Build history of the part. All positions in model axes, mm. A direction names the side the tool comes from. Give positions to 0.01 mm unless a question says otherwise; leave off trailing zeros. Order: outer loops, then holes, each group sorted by start corner. A loop starts at its lowest first (then second) coordinate and runs counter-clockwise, first axis right, second up. Notation, with made-up numbers: M 84,30.25 L 133,30.25 A23 ccw 133,58.25 Z; hole C -16,40 d10. An arc over 180 degrees is marked long. Answer as CSV lines item,"result".
from build123d import *

# Parameters (mm, degrees)
SKETCH_1_W          = 40
SKETCH_1_H          = 20
EXTRUDE_1_DEPTH     = 37
SKETCH_2_W          = 54
SKETCH_2_H          = 20
EXTRUDE_2_DEPTH     = 2.5
SKETCH_3_R          = 2.2
CUT_EXTRUDE_1_DEPTH = 2.5
SKETCH_5_W          = 1.5
SKETCH_5_H          = 2.2
CUT_EXTRUDE_2_DEPTH = 2.5
FILLET_1_R          = 2
EXTRUDE_3_DEPTH     = 2
SKETCH_7_R          = 7.5
EXTRUDE_4_DEPTH     = 1.5
SKETCH_8_R          = 5.5
EXTRUDE_5_DEPTH     = 0.5
SKETCH_9_R          = 3
EXTRUDE_6_DEPTH     = 4
SKETCH_10_R         = 1.5
CUT_EXTRUDE_3_DEPTH = 5


with BuildPart() as part:
    # 草图1 → 凸台-拉伸1 (new body)
    with BuildSketch(Plane(origin=(0, 0, 0), x_dir=(1, 0, 0), z_dir=(0, 1, 0))):
        Rectangle(SKETCH_1_W, SKETCH_1_H)
    extrude(amount=EXTRUDE_1_DEPTH)

    # 草图2 → 凸台-拉伸2 (add)
    with BuildSketch(Plane(origin=(0, 29, 0), x_dir=(-1, 0, 0), z_dir=(0, -1, 0))):
        Rectangle(SKETCH_2_W, SKETCH_2_H)
    extrude(amount=-EXTRUDE_2_DEPTH)

    # 草图3 → 切除-拉伸1 (cut)
    with BuildSketch(Plane(origin=(0, 29, 0), x_dir=(-1, 0, 0), z_dir=(0, -1, 0))):
        with Locations(Location((24.2, 5, 0), (0, 0, 90))):
            Circle(SKETCH_3_R)
        with Locations(Location((-24.2, 5, 0), (0, 0, 90))):
            Circle(SKETCH_3_R)
        with Locations(Location((24.2, -5, 0), (0, 0, 90))):
            Circle(SKETCH_3_R)
        with Locations(Location((-24.2, -5, 0), (0, 0, 90))):
            Circle(SKETCH_3_R)
    extrude(amount=-CUT_EXTRUDE_1_DEPTH, mode=Mode.SUBTRACT)

    # 草图5 → 切除-拉伸2 (cut)
    with BuildSketch(Plane(origin=(0, 29, 0), x_dir=(-1, 0, 0), z_dir=(0, -1, 0))):
        with Locations((-26.25, 5)):
            Rectangle(SKETCH_5_W, SKETCH_5_H)
        with Locations((26.25, 5)):
            Rectangle(SKETCH_5_W, SKETCH_5_H)
        with Locations((26.25, -5)):
            Rectangle(SKETCH_5_W, SKETCH_5_H)
        with Locations((-26.25, -5)):
            Rectangle(SKETCH_5_W, SKETCH_5_H)
    extrude(amount=-CUT_EXTRUDE_2_DEPTH, mode=Mode.SUBTRACT)

    # 圆角1
    fillet_1_edges = [part.edges().sort_by_distance(p)[0] for p in [
        (27, 30.25, -10),
        (-27, 30.25, 10),
        (27, 30.25, 10),
        (-27, 30.25, -10),
    ]]
    fillet(fillet_1_edges, radius=FILLET_1_R)

    # 草图6 → 凸台-拉伸3 (add)
    with BuildSketch(Plane(origin=(0, 37, 0), x_dir=(1, 0, 0), z_dir=(0, 1, 0))):
        with BuildLine():
            Line((-10, 9), (15, 9))
            Line((15, 9), (15, -9))
            Line((15, -9), (-10, -9))
            ThreePointArc((-10, -9), (-19, 0), (-10, 9))
        make_face()
    extrude(amount=EXTRUDE_3_DEPTH)

    # 草图7 → 凸台-拉伸4 (add)
    with BuildSketch(Plane(origin=(0, 39, 0), x_dir=(1, 0, 0), z_dir=(0, 1, 0))):
        with Locations(Location((-10, 0, 0), (0, 0, 270))):
            Circle(SKETCH_7_R)
    extrude(amount=EXTRUDE_4_DEPTH)

    # 草图8 → 凸台-拉伸5 (add)
    with BuildSketch(Plane(origin=(0, 40.5, 0), x_dir=(1, 0, 0), z_dir=(0, 1, 0))):
        with Locations(Location((-10, 0, 0), (0, 0, 270))):
            Circle(SKETCH_8_R)
    extrude(amount=EXTRUDE_5_DEPTH)

    # 草图9 → 凸台-拉伸6 (add)
    with BuildSketch(Plane(origin=(0, 41, 0), x_dir=(1, 0, 0), z_dir=(0, 1, 0))):
        with Locations(Location((-10, 0, 0), (0, 0, 270))):
            Circle(SKETCH_9_R)
    extrude(amount=EXTRUDE_6_DEPTH)

    # 草图10 → 切除-拉伸3 (cut)
    with BuildSketch(Plane(origin=(0, 45, 0), x_dir=(1, 0, 0), z_dir=(0, 1, 0))):
        with Locations(Location((-10, 0, 0), (0, 0, 270))):
            Circle(SKETCH_10_R)
    extrude(amount=-CUT_EXTRUDE_3_DEPTH, mode=Mode.SUBTRACT)


solid = part.part
Item 1: 3-axis set-ups, long thin cutter, end or side, ignore diameter. For faces 1 (the cylindrical face through (-17.32, 39.74, -1.63)), 2 (the flat face through (15, 38, 0)), 3 (the cylindrical face through (-22, 30, -5)): which of +Z, -Z, +X, -X, +Y, -Y reach the whole face in a straight line?
Geometry says:
face 1,"+Y"
face 2,"+Z, -Z, +X, +Y"
face 3,"+Y, -Y"
Item 2: Pull direction Z, two halves, no side cores. Call faces 4 (the cylindrical face through (26.43, 30.27, 9.4)), 5 (the cylindrical face through (22, 30, -5)), 6 (the flat face through (-27, 30, 0)): released by +Z, released by -Z, zero draft, split by the parting line, or undercut.
Geometry says:
face 4,"released by +Z"
face 5,"undercut"
face 6,"zero draft"
Item 3: Band-saw the part on B-B (x = 0). Give the cut face in (y, z), and give its area (3 significant figures).
Geometry says:
outline,"M 0,-10 L 37,-10 L 37,-9 L 39,-9 L 39,9 L 37,9 L 37,10 L 0,10 Z"
area,"776 mm2"
Item 4: Band-saw the part on A-A (x = -24.2). Give the cut face in (y, z), and give its area (3 significant figures).
Geometry says:
outline,"M 29,-10 L 31.5,-10 L 31.5,-7.2 L 29,-7.2 Z; M 29,-2.8 L 31.5,-2.8 L 31.5,2.8 L 29,2.8 Z; M 29,7.2 L 31.5,7.2 L 31.5,10 L 29,10 Z"
area,"28.0 mm2"
Item 5: Probe line 1 along Z through (x, y) = (24, 30); line 2 along X through (y, z) = (43.3, 0); line 3 along X through (y, z) = (29.9, -5). List the from-to ranges inside material, lowest first. Write a range as from..to.
Geometry says:
line 1,"z = -10..-7.19, -2.81..2.81, 7.19..10"
line 2,"x = -13..-11.5, -8.5..-7"
line 3,"x = -22..22"
Item 6: Drop flat-ended pins along their axis: pin 1 (6 mm diameter, centred on y = 14.5, z = 6.5, fed in from -X); pin 2 (6 mm diameter, centred on y = 35, z = -2, fed in from +X); pin 3 (1 mm diameter, centred on x = 3, y = 38, fed in from +Z); pin 4 (2.5 mm diameter, centred on x = 24.2, z = 5, fed in from +Y). Give the stop position or say it passes through.
Geometry says:
pin 1,"stops at x = -20"
pin 2,"stops at x = 20"
pin 3,"stops at z = 9"
pin 4,"passes through"
Item 7: Band-saw the part on D-D (y = 42). Give the cut face in (x, z).
Geometry says:
outline,"C -10,0 d6; hole C -10,0 d3"
